from build123d import *

# Parameters (mm, degrees)
PAD_DEPTH       = 3
SKETCH001_R     = 1.5
POCKET_DEPTH    = 5
SKETCH002_W     = 104
SKETCH002_H     = 34
PAD001_DEPTH    = 40
THICKNESS_T     = -2
POCKET001_DEPTH = 5
SKETCH003_R     = 3
SKETCH003_W     = 8
SKETCH003_H     = 3
POCKET002_DEPTH = 5
SKETCH004_W     = 14
SKETCH004_H     = 2
POCKET003_DEPTH = 5


with BuildPart() as part:
    # Sketch → Pad (new body)
    with BuildSketch(Plane.XY):
        Polygon((-50, 15), (-50, -15), (50, -15), (50, 14.99989), align=None)
    extrude(amount=PAD_DEPTH)

    # Sketch001 (on Face6 of Pad) → Pocket (cut)
    with BuildSketch(Plane.XY.offset(3)):
        with Locations((-47, 12)):
            Circle(SKETCH001_R)
        with Locations((-47, -12)):
            Circle(SKETCH001_R)
        with Locations((0, 11.99989)):
            Circle(SKETCH001_R)
        with Locations((0, -12)):
            Circle(SKETCH001_R)
        with Locations((7, 11.99989)):
            Circle(SKETCH001_R)
        with Locations((7, -12)):
            Circle(SKETCH001_R)
        with Locations((36, 11.99989)):
            Circle(SKETCH001_R)
        with Locations((36, -12)):
            Circle(SKETCH001_R)
    extrude(amount=-POCKET_DEPTH, mode=Mode.SUBTRACT)

    # Sketch002 → Pad001 (join)
    with BuildSketch(Plane.XY):
        Rectangle(SKETCH002_W, SKETCH002_H)
    extrude(amount=PAD001_DEPTH)

    # Thickness
    thickness_openings = [part.faces().sort_by_distance(p)[0] for p in [
        (0, 0, 40),
    ]]
    offset(amount=THICKNESS_T, openings=thickness_openings)

    # Sketch001 (on Face6 of Pad) → Pocket001 (cut)
    with BuildSketch(Plane.XY.offset(3)):
        with Locations((-47, 12)):
            Circle(SKETCH001_R)
        with Locations((-47, -12)):
            Circle(SKETCH001_R)
        with Locations((0, 11.99989)):
            Circle(SKETCH001_R)
        with Locations((0, -12)):
            Circle(SKETCH001_R)
        with Locations((7, 11.99989)):
            Circle(SKETCH001_R)
        with Locations((7, -12)):
            Circle(SKETCH001_R)
        with Locations((36, 11.99989)):
            Circle(SKETCH001_R)
        with Locations((36, -12)):
            Circle(SKETCH001_R)
    extrude(amount=-POCKET001_DEPTH, mode=Mode.SUBTRACT)

    # Sketch003 (on Face1 of Pocket001) → Pocket002 (cut)
    with BuildSketch(Plane(origin=(-52, 0, 0), x_dir=(0, -1, 0), z_dir=(-1, 0, 0))):
        with Locations((0, 17)):
            Circle(SKETCH003_R)
        with Locations((0, 5.5)):
            Rectangle(SKETCH003_W, SKETCH003_H)
    extrude(amount=-POCKET002_DEPTH, mode=Mode.SUBTRACT)

    # Sketch004 (on Face11 of Pocket002) → Pocket003 (cut)
    with BuildSketch(Plane.YZ.offset(52)):
        with Locations((0, 29)):
            Rectangle(SKETCH004_W, SKETCH004_H)
    extrude(amount=-POCKET003_DEPTH, mode=Mode.SUBTRACT)


solid = part.part
Could you check a few things on this model? Use its own coordinates, in mm. A direction names the side the tool comes from. Give positions to 0.01 mm unless a question says otherwise; leave off trailing zeros. Order: outer loops, then holes, each group sorted by start corner. A loop starts at its lowest first (then second) coordinate and runs counter-clockwise, first axis right, second up. Notation, with made-up numbers: (-27, 87.25) -> (13, 87.25) arc R8 cw to (13, 102.25) -> close; hole circle Ø3 at (79, 71.5). An arc over 180 degrees is marked (long way). Answer in a Markdown table with one row per item. Add a question column.
Item 1: Imagine slicing it at C-C (z = 35.5). List the corners of the cut face in (x, y) for me, and give its area (3 significant figures).
Item 2: For faces 1 (the flat face through (51, 7, 29)), 2 (the flat face through (50, 0, 21)), 3 (the flat face through (-51, -4, 5)), which set-ups out of +Z, -Z, +X, -X, +Y, -Y let a thin tool reach every point of the face, with its end or its side?
Item 3: Imagine slicing it at A-A (x = 0). List the corners of the cut face in (y, z) for me, and give its area (3 significant figures).
Item 4: Please list where these lines run through material, in increasing order: probe 1 along Y at (x, z) = (36, 0.9); probe 2 along X at (y, z) = (-10.5, 26.5); probe 3 along Y at (x, z) = (-43.5, 30.5).
Item 5: We'd pull the mould along Z, two halves only. Please class faces 4 (the flat face through (-1, 0, 2)), 5 (the cylindrical face through (-0.325, -13.464, 1.014)), 6 (the cylindrical face through (-51.01, 0.65, 14.07)): pulls with the +Z half, pulls with the -Z half, needs draft (parallel to the pull), parting line crosses it, or undercut.
Item 6: I'm going to push flat-ended pins straight in: P1, Ø2.5, axis at x = -47, y = -12, coming from the -Z side; P2, Ø3.5, axis at y = 0, z = 17, coming from the -X side; P3, Ø3.5, axis at x = 36, y = 12, coming from the +Z side. Where does each tip first touch, or does it pass through?
Item 7: Imagine slicing it at B-B (y = 0). List the corners of the cut face in (x, z) for me, and give its area (3 significant figures).
Item 8: Imagine slicing it at D-D (x = -44.5). List the corners of the cut face in (y, z) for me, and give its area (3 significant figures).
Result:
| question | item | result |
|---|---|---|
| 1 | outline | (-52, -17) -> (52, -17) -> (52, 17) -> (-52, 17) -> close; hole (-50, -15) -> (50, -15) -> (50, 15) -> (-50, 15) -> close |
| 1 | area | 536 mm2 |
| 2 | face 1 | +X |
| 2 | face 2 | +Z |
| 2 | face 3 | -X |
| 3 | outline | (-17, 0) -> (-13.5, 0) -> (-13.5, 2) -> (-15, 2) -> (-15, 40) -> (-17, 40) -> close; (-10.5, 0) -> (10.5, 0) -> (10.5, 2) -> (-10.5, 2) -> close; (13.5, 0) -> (17, 0) -> (17, 40) -> (15, 40) -> (15, 2) -> (13.5, 2) -> close |
| 3 | area | 208 mm2 |
| 4 | probe 1 | -17 to -13.5, -10.5 to 10.5, 13.5 to 17 |
| 4 | probe 2 | -52 to -50, 50 to 52 |
| 4 | probe 3 | -17 to -15, 15 to 17 |
| 5 | face 4 | pulls with the +Z half |
| 5 | face 5 | needs draft |
| 5 | face 6 | undercut |
| 6 | P1 | through |
| 6 | P2 | x = 50 |
| 6 | P3 | z = 2 |
| 7 | outline | (-52, 0) -> (52, 0) -> (52, 28) -> (50, 28) -> (50, 2) -> (-50, 2) -> (-50, 4) -> (-52, 4) -> close; (-52, 7) -> (-50, 7) -> (-50, 14) -> (-52, 14) -> close; (-52, 20) -> (-50, 20) -> (-50, 40) -> (-52, 40) -> close; (50, 30) -> (52, 30) -> (52, 40) -> (50, 40) -> close |
| 7 | area | 338 mm2 |
| 8 | outline | (-17, 0) -> (17, 0) -> (17, 40) -> (15, 40) -> (15, 2) -> (-15, 2) -> (-15, 40) -> (-17, 40) -> close |
| 8 | area | 220 mm2 |
